Source: CAD feature listing. Evaluate the final solid. Frame: model axes, mm. A direction names the side the tool comes from. Round coordinates to 2 decimals unless told otherwise and drop trailing zeros. Loops run counter-clockwise (first coordinate to the right, second up) from the corner with the lowest first, then second, coordinate; pieces in that order, holes last. Notation, with made-up numbers: (52, -4) -> (87, -4) arc R19 ccw to (87, 23) -> close; hole circle Ø5 at (-36.75, -26). An arc over 180 degrees is marked (long way). Put each result on its own line as item: value. Start each with the question number.
1. Cut plane A-A (y = 0). State how many separate pieces and enclosed holes the cut face has, then the cut area to 3 significant figures.
2. Set-up query: faces 1 (the flat face through (69.85, 2, 3)), 2 (the cylindrical face through (-0.1, 3.9, 3.2)). Return all of +Z, -Z, +X, -X, +Y, -Y with unobstructed straight access to the full face (end or side cutting, diameter ignored); none if empty.
3. Cut plane B-B (x = 0). Return the cut outline in (y, z), then the cut area to 3 significant figures.
4. Cut plane C-C (x = -57.5). Return the cut outline in (y, z).
5. Material intervals for L1, parallel to X at y = -4.25, z = 3 (3 decimals); L2, parallel to X at y = 0.5, z = 3.25; L3, parallel to X at y = -3, z = 4.25, sorted ascending.
6. Draft query along X for faces 3 (the flat face through (-76, -3.175, 5)), 4 (the flat face through (-79.375, -5, 3)), 5 (the cylindrical face through (58.6, 3.9, 3.2)). Return one class per face: pulls with the +X half, pulls with the -X half, needs draft (parallel to the pull), parting line crosses it, or undercut.
7. Contact query for flat-ended pins moving along their axis: pin 1 (5 mm diameter, centred on x = 20, y = -0.5, fed in from -Z); pin 2 (1 mm diameter, centred on y = -0.5, z = 5, fed in from -X); pin 3 (1.9 mm diameter, centred on x = 76.5, z = 2.5, fed in from +Y) (3 decimals). Output: stop coordinate, or through.
```python
from build123d import *

# Parameters (mm, degrees)
SKETCH1_W                   = 139.7
SKETCH1_H                   = 12.7
BOSS_EXTRUDE1_DEPTH         = 6.35
SKETCH2_R                   = 2.4511
CUT_EXTRUDE1_DEPTH          = 7.35
TAP_DRILL_FOR_M3X0_5_TAP1_D = 2.5
SKETCH5_W                   = 9.525
SKETCH5_H                   = 6.35
BOSS_EXTRUDE2_DEPTH         = 3.175
FILLET1_R                   = 1.5875
M3_CLEARANCE_HOLE1_D        = 3.4
FILLET2_R                   = 1.5875
FILLET2_OF_MIRROR5_R        = 1.5875
FILLET3_R                   = 1.5875


with BuildPart() as part:
    # Sketch1 → Boss-Extrude1 (new body)
    with BuildSketch(Plane.XY):
        Rectangle(SKETCH1_W, SKETCH1_H)
    extrude(amount=BOSS_EXTRUDE1_DEPTH)

    # Sketch2 → Cut-Extrude1 (cut, through all)
    with BuildSketch(Plane.XY.offset(6.35)):
        with Locations((0, 6.35)):
            Circle(SKETCH2_R)
        with Locations((5.334, 6.35)):
            Circle(SKETCH2_R)
        with Locations((10.668, 6.35)):
            Circle(SKETCH2_R)
        with Locations((16.002, 6.35)):
            Circle(SKETCH2_R)
        with Locations((21.336, 6.35)):
            Circle(SKETCH2_R)
        with Locations((26.67, 6.35)):
            Circle(SKETCH2_R)
        with Locations((32.004, 6.35)):
            Circle(SKETCH2_R)
        with Locations((37.338, 6.35)):
            Circle(SKETCH2_R)
        with Locations((42.672, 6.35)):
            Circle(SKETCH2_R)
        with Locations((48.006, 6.35)):
            Circle(SKETCH2_R)
        with Locations((53.34, 6.35)):
            Circle(SKETCH2_R)
        with Locations((58.674, 6.35)):
            Circle(SKETCH2_R)
        with Locations((-5.334, 6.35)):
            Circle(SKETCH2_R)
        with Locations((-10.668, 6.35)):
            Circle(SKETCH2_R)
        with Locations((-16.002, 6.35)):
            Circle(SKETCH2_R)
        with Locations((-21.336, 6.35)):
            Circle(SKETCH2_R)
        with Locations((-26.67, 6.35)):
            Circle(SKETCH2_R)
        with Locations((-32.004, 6.35)):
            Circle(SKETCH2_R)
        with Locations((-37.338, 6.35)):
            Circle(SKETCH2_R)
        with Locations((-42.672, 6.35)):
            Circle(SKETCH2_R)
        with Locations((-48.006, 6.35)):
            Circle(SKETCH2_R)
        with Locations((-53.34, 6.35)):
            Circle(SKETCH2_R)
        with Locations((-58.674, 6.35)):
            Circle(SKETCH2_R)
    extrude(amount=-CUT_EXTRUDE1_DEPTH, mode=Mode.SUBTRACT)

    # Tap Drill for M3x0.5 Tap1 (through all)
    with Locations(Plane(origin=(0, 6.35, 0), x_dir=(1, 0, 0), z_dir=(0, 1, 0))):
        with Locations((-65.0875, -3.175), (65.0875, -3.175)):
            Hole(TAP_DRILL_FOR_M3X0_5_TAP1_D / 2)

    # Sketch5 → Boss-Extrude2 (add)
    with BuildSketch(Plane.XZ.offset(6.35)):
        with Locations((-74.6125, 3.175)):
            Rectangle(SKETCH5_W, SKETCH5_H)
    boss_extrude2 = extrude(amount=-BOSS_EXTRUDE2_DEPTH)

    # Fillet1
    fillet1_edges = [part.edges().sort_by_distance(p)[0] for p in [
        (-69.85, -3.175, 3.175),
    ]]
    fillet(fillet1_edges, radius=FILLET1_R)

    # M3 Clearance Hole1 (through all)
    with Locations(Plane(origin=(0, -3.175, 0), x_dir=(1, 0, 0), z_dir=(0, 1, 0))):
        with Locations((-75.40625, -3.175)):
            m3_clearance_hole1 = Hole(M3_CLEARANCE_HOLE1_D / 2)

    # Fillet2
    fillet2_edges = [part.edges().sort_by_distance(p)[0] for p in [
        (-79.375, -4.7625, 0),
        (-79.375, -4.7625, 6.35),
    ]]
    fillet(fillet2_edges, radius=FILLET2_R)

    # Mirror5: Boss-Extrude2, M3 Clearance Hole1 across plane
    add(boss_extrude2.mirror(Plane(origin=(0, 0, 0), x_dir=(0, 0, 1), z_dir=(1, 0, 0))))
    add(m3_clearance_hole1.mirror(Plane(origin=(0, 0, 0), x_dir=(0, 0, 1), z_dir=(1, 0, 0))), mode=Mode.SUBTRACT)

    # Fillet2 of Mirror5
    fillet2_of_mirror5_edges = [part.edges().sort_by_distance(p)[0] for p in [
        (79.375, -4.7625, 0),
        (79.375, -4.7625, 6.35),
    ]]
    fillet(fillet2_of_mirror5_edges, radius=FILLET2_OF_MIRROR5_R)

    # Fillet3
    fillet3_edges = [part.edges().sort_by_distance(p)[0] for p in [
        (69.85, -3.175, 3.175),
    ]]
    fillet(fillet3_edges, radius=FILLET3_R)


solid = part.part
```
Solution:
1. separate pieces: 1
1. enclosed holes: 2
1. area: 877 mm^2
2. face 1: +Z, -Z, +X, +Y
2. face 2: +Z, -Z, +Y
3. outline: (-6.35, 0) -> (3.9, 0) -> (3.9, 6.35) -> (-6.35, 6.35) -> close
3. area: 65.1 mm^2
4. outline: (-6.35, 0) -> (4.2, 0) -> (4.2, 6.35) -> (-6.35, 6.35) -> close
5. L1: x = -79.375 to -77.097, -73.715 to -66.325, -63.85 to 63.85, 66.325 to 73.715, 77.097 to 79.375
5. L2: x = -69.85 to -66.34, -63.84 to 63.84, 66.34 to 69.85
5. L3: x = -70.71 to -65.73, -64.45 to 64.45, 65.73 to 70.71
6. face 3: needs draft
6. face 4: pulls with the -X half
6. face 5: undercut
7. pin 1: stops at z = 0
7. pin 2: stops at x = -69.85
7. pin 3: stops at y = -3.175
